from build123d import *

# Parameters (mm, degrees)
SKETCH2_R           = 3.175
BOSS_EXTRUDE1_DEPTH = 22.098
SKETCH3_W           = 6.414942463
SKETCH3_H           = 22.098
BOSS_EXTRUDE2_DEPTH = 6.35
SKETCH5_W           = 18.491886748
SKETCH5_H           = 65.278
SKETCH5_R           = 3.175
BOSS_EXTRUDE4_DEPTH = 5.08
BOSS_EXTRUDE7_REACH = 239.969
SKETCH7_W           = 22.098
SKETCH7_H           = 24.955967439


with BuildPart() as part:
    # Sketch2 → Boss-Extrude1 (new body)
    with BuildSketch(Plane.XY):
        Polygon((-633.396746705, 209.866473294), (-629.456250373, 228.608305414), (-646.417262265, 232.174381811), (-650.357758597, 213.432549691), align=None)
        with Locations(Location((-637.11116423, 215.213960129, 0), (0, 0, 180))):
            Circle(SKETCH2_R, mode=Mode.SUBTRACT)
        with Locations(Location((-635.053635704, 225, 0), (0, 0, 180))):
            Circle(SKETCH2_R, mode=Mode.SUBTRACT)
    extrude(amount=BOSS_EXTRUDE1_DEPTH)

    # Sketch3 → Boss-Extrude2 (add)
    with BuildSketch(Plane(origin=(15.442364745, 73.44714554, 0), x_dir=(0.9786039871389689, -0.20575285260650172, 0), z_dir=(-0.20575285260650172, -0.9786039871389689, 0))):
        with Locations((-677.149580337, 11.049)):
            Rectangle(SKETCH3_W, SKETCH3_H)
    extrude(amount=BOSS_EXTRUDE2_DEPTH)

    # Sketch5 → Boss-Extrude4 (add)
    with BuildSketch(Plane(origin=(0, 207.218414372, 0), x_dir=(1, 0, 0), z_dir=(0, 1, 0))):
        with Locations((-648.768345837, -11.049)):
            Rectangle(SKETCH5_W, SKETCH5_H)
        with Locations(Location((-648.793402463, -33.528, 0), (0, 0, 270))):
            Circle(SKETCH5_R, mode=Mode.SUBTRACT)
        with Locations(Location((-648.793402463, 11.43, 0), (0, 0, 270))):
            Circle(SKETCH5_R, mode=Mode.SUBTRACT)
    extrude(amount=-BOSS_EXTRUDE4_DEPTH)

    # Boss-Extrude7: up to this face of the body (flat: up to its plane)
    boss_extrude7_end = Plane(part.part.faces().sort_by_distance((-649.040775738, 219.696398091, 11.049))[0])
    # Sketch7 → Boss-Extrude7 (add, up to the picked face)
    with BuildSketch(Plane.ZY.offset(658.014289211), mode=Mode.PRIVATE) as boss_extrude7_sk1:
        with Locations((11.049, 219.696398092)):
            Rectangle(SKETCH7_W, SKETCH7_H)
    boss_extrude7_tool1 = split(extrude(boss_extrude7_sk1.sketch, amount=-BOSS_EXTRUDE7_REACH, mode=Mode.PRIVATE), bisect_by=boss_extrude7_end, keep=Keep.BOTH, mode=Mode.PRIVATE)
    add(boss_extrude7_tool1.solids().sort_by(Axis((-658.014289, 219.696398, 11.049), (1, 0, 0)))[0])


solid = part.part
Can you work these out from the model? Positions are in its coordinate system, mm. A direction names the side the tool comes from. Coordinates: 2 decimals unless noted, no trailing zeros. Order: outer loops, then holes, each group sorted by start corner. A loop starts at its lowest first (then second) coordinate and runs counter-clockwise, first axis right, second up. Notation, with made-up numbers: (34, 33.5) - (93, 33.5) arc R7 cw to (93, 43.5) - close; hole circle Ø7 at (-13.5, 62). An arc over 180 degrees is marked (long way). Answer as a JSON object with one key per item and string values. Group by question number.
Q1. On a 3-axis mill with a long thin cutter (end or side, diameter ignored), from which of +Z, -Z, +X, -X, +Y, -Y can I reach the whole of each face in a straight line? I mean faces 1 (the face through (-647, 220, 0)), 2 (the face through (-644.8, 207.218, 10.6)), 3 (the face through (-639.522, 205, 12)), 4 (the face through (-638.813, 211.005, 10.894)). Say none if no direction works.
Q2. Will these pins go through, and if not, where does the flat tip stop? P1, Ø6, axis at x = -655, y = 220, coming from the +Z side; P2, Ø8.5, axis at x = -635.05, y = 225, coming from the -Z side; P3, Ø1.5, axis at y = 205, z = 12.5, coming from the +X side.
Q3. Imagine slicing it at D-D (x = -655). Please give me the cut outline in (y, z), and give its area (3 significant figures).
Q4. Imagine slicing it at A-A (z = -11.43). Please give me the cut outline in (x, y).
Q5. Imagine slicing it at C-C (y = 223.5). Please give me the cut outline in (x, z).
Q6. We'd pull the mould along Y, two halves only. Please class faces 5 (the face through (-644.587, 209.7, 10.894)), 6 (the face through (-652, 232.174, 11)), 7 (the face through (-645.645, 204.714, -11.843)): +Y half, -Y half, draft (parallel to the pull), parting line (faces both ways), or undercut.
Q7. Imagine slicing it at B-B (x = -649.75). Please give me the cut outline in (y, z).
Q8. I need wall thicknesses on line 1 (X direction, y = 205.1, z = -11.43); line 2 (Y direction, x = -644.5, z = -5.5); line 3 (Z direction, x = -642.5, y = 213). Which ranges of each line are inside material? Lowest first, please. Write a range as from..to.
Determined:
{
 "1": {"face 1": "-Z, +X, -X, +Y", "face 2": "+X", "face 3": "+Z, -Z, +X, -Y", "face 4": "+Z, -Z"},
 "2": {"P1": "stops at z = 22.1", "P2": "stops at z = 0", "P3": "stops at x = -639.52"},
 "3": {"outline": "(202.14, -21.59) - (207.22, -21.59) - (207.22, 0) - (232.17, 0) - (232.17, 22.1) - (207.22, 22.1) - (207.22, 43.69) - (202.14, 43.69) - close", "area": "883 mm2"},
 "4": {"outline": "(-658.01, 202.14) - (-651.97, 202.14) - (-651.97, 207.22) - (-658.01, 207.22) - close; (-645.62, 202.14) - (-639.52, 202.14) - (-639.52, 207.22) - (-645.62, 207.22) - close"},
 "5": {"outline": "(-658.01, 0) - (-637.85, 0) - (-637.85, 22.1) - (-658.01, 22.1) - close; (-632.26, 0) - (-630.53, 0) - (-630.53, 22.1) - (-632.26, 22.1) - close"},
 "6": {"face 5": "undercut", "face 6": "+Y half", "face 7": "draft"},
 "7": {"outline": "(202.14, -21.59) - (207.22, -21.59) - (207.22, -14.46) - (202.14, -14.46) - close; (202.14, -8.4) - (207.22, -8.4) - (207.22, 0) - (232.17, 0) - (232.17, 22.1) - (207.22, 22.1) - (207.22, 30.5) - (202.14, 30.5) - close; (202.14, 36.56) - (207.22, 36.56) - (207.22, 43.69) - (202.14, 43.69) - close"},
 "8": {"line 1": "x = -658.01..-651.97, -645.62..-639.52", "line 2": "y = 202.14..207.22", "line 3": "z = 0..22.1"}
}
